Part model, mm, in its own coordinate system. Face numbers are marked on the shaded views. A direction names the side the tool comes from. Round coordinates to 2 decimals unless told otherwise and drop trailing zeros. Write each loop counter-clockwise with the first axis right and the second up, starting at its lowest first coordinate (ties: lowest second). Pieces come first, ordered by that corner, then holes. Notation, with made-up numbers: (-5, 32.5) -> (36, 32.5) arc R33 ccw to (36, 60.5) -> close; hole circle Ø11 at (-11, -40). An arc over 180 degrees is marked (long way). Return JSON: item names as keys, results as strings. Group by question number.
(1) Tool access for the marked faces 1 and 2: list every direction of +Z, -Z, +X, -X, +Y, -Y with a clear straight run to the whole face (end or side of a thin tool).
(2) Drill centre lines: L1, parallel to Y at x = 2.5, z = 1.5; L2, parallel to X at y = -2.5, z = 1; L3, parallel to X at y = -2, z = 0. Where is each one in solid material? Low to high. Write a range as from..to.
(3) Drop flat-ended pins along their axis: pin 1 Ø1.6 at (x, y) = (-2, -2.5) entering from +Z; pin 2 Ø2 at (x, z) = (-3, 3) entering from -Y; pin 3 Ø3.5 at (x, z) = (1, 3.5) entering from +Y; pin 4 Ø1.1 at (x, y) = (1, -2) entering from -Z. Give the stop position or say it passes through.
(4) Mould opens along Z. For the marked faces 3, 4 and 5 say: +Z half, -Z half, draft (parallel to the pull), parting line (faces both ways), or undercut.
(5) Saw through at A-A (y = 5.25). List the corners of the cut face in (x, z), plus the area to 3 significant figures.
from build123d import *

# Parameters (mm, degrees)
FILLET_1_R          = 0.5
CUT_EXTRUDE_1_DEPTH = 1.5


with BuildPart() as part:
    # 草图2 → 旋转1 (revolve)
    with BuildSketch(Plane(origin=(0, 0, 0), x_dir=(0, 0, -1), z_dir=(1, 0, 0))):
        with BuildLine():
            Line((1.817800027, -0.459726703), (-0.182199973, -0.459726703))
            Line((-0.182199973, -0.459726703), (-0.182199973, 7.540273297))
            Line((-0.182199973, 7.540273297), (-1.682199973, 7.540273297))
            Line((-1.682199973, 7.540273297), (-1.682199973, -0.459726703))
            Line((-1.682199973, -0.459726703), (-1.682199973, -2.959726703))
            add(Edge.make_bspline(
                [(1.817800027, -1.252007585), (1.177768259, -2.02578844), (0.30662425, -2.840564308), (-1.682199973, -2.959726703)],
                knots=[0, 0, 0, 0, 1, 1, 1, 1], degree=3))
            Line((1.817800027, -1.252007585), (1.817800027, -0.459726703))
        make_face()
    revolve(axis=Axis((0, -0.459726703, 1.682199973), (0, 1, 0)))

    # 圆角1
    fillet_1_edges = [part.edges().sort_by_distance(p)[0] for p in [
        (0, -1.252007585, 5.182199973),
    ]]
    fillet(fillet_1_edges, radius=FILLET_1_R)

    # 草图3 → 切除-拉伸1 (cut)
    with BuildSketch(Plane(origin=(0, -2.959726703, 0), x_dir=(-1, 0, 0), z_dir=(0, -1, 0))):
        Polygon((-0.470758808, -1.182199973), (-2.75, -1.182199973), (-2.75, -2.182199973), (-0.470758808, -2.182199973), (-0.470758808, -4.426883393), (0.529241192, -4.426883393), (0.529241192, -2.182199973), (2.75, -2.182199973), (2.75, -1.182199973), (0.529241192, -1.182199973), (0.529241192, 1.073116607), (-0.470758808, 1.073116607), align=None)
    extrude(amount=-CUT_EXTRUDE_1_DEPTH, mode=Mode.SUBTRACT)


solid = part.part
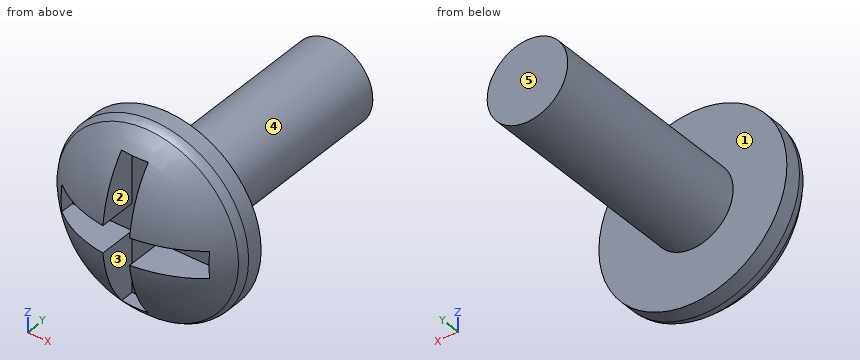
Computed values:
{
 "1": {"face 1": "+Y", "face 2": "-Y"},
 "2": {"L1": "-1.46..-0.46", "L2": "-1.85..-0.53, 0.47..1.85", "L3": "-2.19..-0.53, 0.47..2.19"},
 "3": {"pin 1": "z = 4.2", "pin 2": "y = -2.34", "pin 3": "y = 7.54", "pin 4": "z = -1.52"},
 "4": {"face 3": "undercut", "face 4": "parting line", "face 5": "draft"},
 "5": {"outline": "circle Ø3 at (0, 1.68)", "area": "7.07 mm2"}
}
